Part model, mm, in its own coordinate system. A direction names the side the tool comes from. Coordinates: 2 decimals unless noted, no trailing zeros. Write each loop counter-clockwise with the first axis right and the second up, starting at its lowest first coordinate (ties: lowest second). Pieces come first, ordered by that corner, then holes. Notation, with made-up numbers: M 50.25,-25 L 99.25,-25 A21 cw 99.25,2 Z; hole C 85.5,-29 d5. An arc over 180 degrees is marked long. Use a Markdown table: item, result. Add a question column.
Q1. Slice it at B-B on y = -18. Write the cut outline in (x, z), then the cut area to 3 significant figures.
Q2. Slice it at D-D on x = -6. Write the cut outline in (y, z), then the cut area to 3 significant figures.
Q3. Wall check: L1, parallel to Y at x = 0, z = 3.25; L2, parallel to Y at x = -6.5, z = 3.7; L3, parallel to Y at x = 1, z = 0.75. Give the ranges that are in metal, low to high. Write a range as from..to.
Q4. Mould opens along Y. For faces 1 (the flat face through (4.5, -23, 2)), 2 (the cylindrical face through (15.248, -33.287, 2.028)), 3 (the flat face through (14, 0, 0)) say: released by +Y, released by -Y, zero draft, split by the parting line, or undercut.
Q5. Slice it at C-C on z = 3.1. Write the cut outline in (x, y).
Q6. Tool access for faces 4 (the flat face through (-12, 0, 2)), 5 (the flat face through (0, -34, 2)), 6 (the flat face through (0.1, 24, 2.4)): list every direction of +Z, -Z, +X, -X, +Y, -Y with a clear straight run to the whole face (end or side of a thin tool).
Q7. Slice it at A-A on x = 0. Count the separate pieces of the cut face and the enclosed holes in it, then the cut area to 3 significant figures.
Solid Edge part; units mm, degrees
sketch "Sketch1" plane through (0, 0, 0) normal (0, 0, 1) x (1, 0, 0)
  line L0 (-16, 34) -> (16, 34)
  line L1 (16, 34) -> (16, -34)
  line L2 (16, -34) -> (-16, -34)
  line L3 (-16, -34) -> (-16, 34)
  line L4 (-3, 27.5) -> (3, 27.5)
  line L5 (-3, 30.5) -> (3, 30.5)
  arc A0 (3, 30.5) -> (3, 27.5) centre (3, 29) cw
  arc A1 (-3, 27.5) -> (-3, 30.5) centre (-3, 29) cw
  arc A2 (3, -30.5) -> (3, -27.5) centre (3, -29) ccw
  line L6 (-3, -27.5) -> (3, -27.5)
  arc A3 (-3, -27.5) -> (-3, -30.5) centre (-3, -29) ccw
  line L7 (-3, -30.5) -> (3, -30.5)
  line L8 (-12, 20) -> (12, 20)
  line L9 (12, -20) -> (12, 20)
  line L10 (12, -20) -> (-12, -20)
  line L11 (-12, 20) -> (-12, -20)
extrude "Protrusion1" add sketch "Sketch1" along normal blind 4
sketch "Sketch2" plane through (0, 0, 0) normal (0, 0, 1) x (1, 0, 0)
  line L0 (4.5, 24) -> (-4.5, 24)
  line L1 (-4.5, 24) -> (-4.5, 20)
  line L2 (-4.5, 20) -> (4.5, 20)
  line L3 (4.5, 20) -> (4.5, 24)
extrude "ExtrudedCutout_3" cut sketch "Sketch2" along normal blind 4
fillet "Round_2" radius 2.5 4 edges at (16, 34, 2) (-16, 34, 2) (-16, -34, 2) (16, -34, 2)
sketch "Sketch3" plane through (0, 0, 0) normal (0, 0, 1) x (1, 0, 0)
  line L0 (4.5, -24) -> (-4.5, -24)
  line L1 (-4.5, -24) -> (-4.5, -20)
  line L2 (-4.5, -20) -> (4.5, -20)
  line L3 (4.5, -20) -> (4.5, -24)
extrude "ExtrudedCutout_6" cut sketch "Sketch3" along normal blind 17.8081
sketch "Sketch4" plane through (0, 0, 0) normal (0, 0, -1) x (-1, 0, 0)
  line L0 (4.5, 22) -> (12, 22)
  line L1 (12, 22) -> (12, 20)
  line L2 (12, 20) -> (4.5, 20)
  line L3 (4.5, 20) -> (4.5, 22)
  line L4 (-12, 22) -> (-4.5, 22)
  line L5 (-4.5, 22) -> (-4.5, 20)
  line L6 (-4.5, 20) -> (-12, 20)
  line L7 (-12, 20) -> (-12, 22)
  line L8 (12, -22) -> (4.5, -22)
  line L9 (4.5, -22) -> (4.5, -20)
  line L10 (4.5, -20) -> (12, -20)
  line L11 (12, -20) -> (12, -22)
  line L12 (-12, -20) -> (-4.5, -20)
  line L13 (-4.5, -20) -> (-4.5, -22)
  line L14 (-4.5, -22) -> (-12, -22)
  line L15 (-12, -22) -> (-12, -20)
extrude "ExtrudedCutout_7" cut sketch "Sketch4" against normal blind 14.5789
sketch "Sketch5" plane through (-4.5, 22, 2) normal (0, 0, 1) x (1, 0, 0)
  line L0 (3, 0) -> (6, 0)
  line L1 (6, 0) -> (6, 2)
  line L2 (6, 2) -> (3, 2)
  line L3 (3, 2) -> (3, 0)
  line L4 (3, -44) -> (6, -44)
  line L5 (6, -44) -> (6, -46)
  line L6 (6, -46) -> (3, -46)
  line L7 (3, -46) -> (3, -44)
extrude "Protrusion2" add sketch "Sketch5" against normal up to vertex (2 mm away)
fillet "Round_4" radius 2 2 edges at (0, 22, 2) (0, -22, 2)
Recorded:
| question | item | result |
|---|---|---|
| 1 | outline | M -16,0 L -12,0 L -12,4 L -16,4 Z; M 12,0 L 16,0 L 16,4 L 12,4 Z |
| 1 | area | 32.0 mm² |
| 2 | outline | M -34,0 L -22,0 L -22,4 L -34,4 Z; M 22,0 L 34,0 L 34,4 L 22,4 Z |
| 2 | area | 96.0 mm² |
| 3 | L1 | -34..-30.5, -27.5..-24, 24..27.5, 30.5..34 |
| 3 | L2 | -34..-22, 22..34 |
| 3 | L3 | -34..-30.5, -27.5..-22.15, 22.15..27.5, 30.5..34 |
| 4 | face 1 | undercut |
| 4 | face 2 | released by -Y |
| 4 | face 3 | zero draft |
| 5 | outline | M -16,-31.5 A2.5 ccw -13.5,-34 L 13.5,-34 A2.5 ccw 16,-31.5 L 16,31.5 A2.5 ccw 13.5,34 L -13.5,34 A2.5 ccw -16,31.5 Z; hole M -12,-22 L -4.5,-22 L -4.5,-24 L 4.5,-24 L 4.5,-22 L 12,-22 L 12,22 L 4.5,22 L 4.5,24 L -4.5,24 L -4.5,22 L -12,22 Z; hole M -3,-30.5 L 3,-30.5 A1.5 ccw 3,-27.5 L -3,-27.5 A1.5 ccw Z; hole M -3,27.5 L 3,27.5 A1.5 ccw 3,30.5 L -3,30.5 A1.5 ccw Z |
| 6 | face 4 | +Z, -Z |
| 6 | face 5 | +Z, -Z, +X, -X, -Y |
| 6 | face 6 | +Z |
| 7 | separate pieces | 4 |
| 7 | enclosed holes | 0 |
| 7 | area | 62.3 mm² |
